```python
from build123d import *

# Parameters (mm, degrees)
SKETCH_1_W               = 32
SKETCH_1_H               = 12
F_32X12_3_3MM_DEPTH      = 3
SKETCH_2_W               = 8
SKETCH_2_H               = 27
EXTRUDE_3_DEPTH          = 3
SKETCH_3_R               = 1.8
CUT_EXTRUDE_3_6_27_DEPTH = 3
SKETCH_4_R               = 1.8
CUT_EXTRUDE_832_DEPTH    = 3


with BuildPart() as part:
    # 草图1 → 测距小底脚32x12_厚3_单向3mm (new body)
    with BuildSketch(Plane(origin=(0, 0, 0), x_dir=(1, 0, 0), z_dir=(0, 1, 0))):
        with Locations((0, 3)):
            Rectangle(SKETCH_1_W, SKETCH_1_H)
    extrude(amount=F_32X12_3_3MM_DEPTH)

    # 草图2 → 两根支撑臂厚3_去掉大框和加强筋 (add)
    with BuildSketch(Plane.XY):
        with Locations((-13.5, 16.5)):
            Rectangle(SKETCH_2_W, SKETCH_2_H)
        with Locations((13.5, 16.5)):
            Rectangle(SKETCH_2_W, SKETCH_2_H)
    extrude(amount=EXTRUDE_3_DEPTH)

    # 草图3 → 背板原孔3.6_只接下排两孔距27_贯穿 (cut)
    with BuildSketch(Plane.XY):
        with Locations((-13.5, 25)):
            Circle(SKETCH_3_R)
        with Locations((13.5, 25)):
            Circle(SKETCH_3_R)
    extrude(amount=CUT_EXTRUDE_3_6_27_DEPTH, mode=Mode.SUBTRACT)

    # 草图4 → Cut-Extrude 832 (cut)
    with BuildSketch(Plane(origin=(0, 0, 0), x_dir=(1, 0, 0), z_dir=(0, 1, 0))):
        with Locations(Location((-11, 4.5, 0), (0, 0, 270))):
            Circle(SKETCH_4_R)
        with Locations(Location((11, 4.5, 0), (0, 0, 270))):
            Circle(SKETCH_4_R)
    extrude(amount=CUT_EXTRUDE_832_DEPTH, mode=Mode.SUBTRACT)


solid = part.part
```
For this review, take the finished solid that the model builds, in its own axes (mm). A direction names the side the tool comes from. Coordinates: 2 decimals unless noted, no trailing zeros. Write each loop counter-clockwise with the first axis right and the second up, starting at its lowest first coordinate (ties: lowest second). Pieces come first, ordered by that corner, then holes.
(1) Wall thickness on probe 1 along X at (y, z) = (1, -4.5); probe 2 along Y at (x, z) = (13.5, 1.6); probe 3 along X at (y, z) = (6, 2.5): over which ranges is each line inside the solid? List them lowest first.
(2) Tool access review of faces 1 (the face through (-9.5, 16, 1)), 2 (the face through (-14, 30, 1)), 3 (the face through (17, 3, 1)), 4 (the face through (-16, 1, -3)): name each direction out of +Z, -Z, +X, -X, +Y, -Y from which nothing blocks a thin tool from reaching the whole face with its end or side.
(3) For pin 1 Ø8 at (x, y) = (-10.5, 19) entering from -Z; pin 2 Ø2.5 at (y, z) = (1.5, -1) entering from -X; pin 3 Ø3 at (y, z) = (4, -3) entering from +X, all flat-tipped, find the tip position at first contact; note any pin that passes through.
(4) Add section D-D on y = 25. Give the boundary of the cut face in (x, z).
(5) Add section B-B on z = -4.5. Give the boundary of the cut face in (x, y).
(6) Add section A-A on y = 9.25. Give the boundary of the cut face in (x, z), then the cut area to 3 significant figures.
(7) Add section C-C on x = -13.5. Give the boundary of the cut face in (y, z), then the cut area to 3 significant figures.
(8) The part is to be moulded in two halves that separate along Z. For faces 5 (the face through (13, 17, 0)), 6 (the face through (13.266, 26.785, 1.479)), 7 (the face through (10.311, 1.479, -2.837)), say which applies: +Z half, -Z half, draft (parallel to the pull), parting line (faces both ways), or undercut.
Answer sheet:
1. probe 1: x = -16 to -12.8, -9.2 to 9.2, 12.8 to 16
1. probe 2: y = 0 to 23.2, 26.8 to 30
1. probe 3: x = -17.5 to -9.5, 9.5 to 17.5
2. face 1: +Z, -Z, +Y
2. face 2: +Z, -Z, +X, -X, +Y
2. face 3: +Z, -Z, +X, -Y
2. face 4: +Z, -Z, -X, -Y
3. pin 1: stops at z = 0
3. pin 2: stops at x = -16
3. pin 3: stops at x = 16
4. outline: (-17.5, 0) - (-15.3, 0) - (-15.3, 3) - (-17.5, 3) - close; (-11.7, 0) - (-9.5, 0) - (-9.5, 3) - (-11.7, 3) - close; (9.5, 0) - (11.7, 0) - (11.7, 3) - (9.5, 3) - close; (15.3, 0) - (17.5, 0) - (17.5, 3) - (15.3, 3) - close
5. outline: (-16, 0) - (-12.8, 0) - (-12.8, 3) - (-16, 3) - close; (-9.2, 0) - (9.2, 0) - (9.2, 3) - (-9.2, 3) - close; (12.8, 0) - (16, 0) - (16, 3) - (12.8, 3) - close
6. outline: (-17.5, 0) - (-9.5, 0) - (-9.5, 3) - (-17.5, 3) - close; (9.5, 0) - (17.5, 0) - (17.5, 3) - (9.5, 3) - close
6. area: 48.0 mm2
7. outline: (0, -9) - (3, -9) - (3, 0) - (23.2, 0) - (23.2, 3) - (0, 3) - close; (26.8, 0) - (30, 0) - (30, 3) - (26.8, 3) - close
7. area: 106 mm2
8. face 5: -Z half
8. face 6: draft
8. face 7: undercut
